```python
from build123d import *

# Parameters (mm, degrees)
BOSS_EXTRUDE1_DEPTH = 50
CUT_EXTRUDE1_DEPTH  = 50


with BuildPart() as part:
    # Sketch2 → Boss-Extrude1 (new body)
    with BuildSketch(Plane.XY):
        with BuildLine():
            Line((-133.871822526, 14.839434035), (-58.871822526, 14.839434035))
            Line((-58.871822526, 14.839434035), (15.717319626, 22.67906878))
            Line((15.717319626, 22.67906878), (16.762604259, 12.733849826))
            Line((16.762604259, 12.733849826), (-48.921026621, 5.830222033))
            ThreePointArc((-48.921026621, 5.830222033), (-58.375818015, -5.148257366), (-68.871822526, 4.839434035))
            Line((-68.871822526, 4.839434035), (-133.871822526, 4.839434035))
            Line((-133.871822526, 4.839434035), (-133.871822526, 14.839434035))
        make_face()
    extrude(amount=BOSS_EXTRUDE1_DEPTH)

    # Sketch4 → Cut-Extrude1 (cut)
    with BuildSketch(Plane.XY.offset(50)):
        with BuildLine():
            Line((-68.871822526, 0.839434035), (-68.871822526, 4.839434035))
            ThreePointArc((-68.871822526, 4.839434035), (-66.871822526, 2.839434035), (-68.871822526, 0.839434035))
        make_face()
        with BuildLine():
            Line((-48.502912768, 1.852134452), (-48.921026621, 5.830222033))
            ThreePointArc((-48.921026621, 5.830222033), (-50.701013486, 3.632121316), (-48.502912768, 1.852134452))
        make_face()
    extrude(amount=-CUT_EXTRUDE1_DEPTH, mode=Mode.SUBTRACT)


solid = part.part
```
Input: part model. Units: mm. Frame: model coordinates. A direction names the side the tool comes from. Coordinates: 2 decimals unless noted, no trailing zeros. Write each loop counter-clockwise with the first axis right and the second up, starting at its lowest first coordinate (ties: lowest second). Pieces come first, ordered by that corner, then holes. Notation, with made-up numbers: (79, 62) -> (106, 62) arc R14 cw to (106, 82) -> close; hole circle Ø10 at (-32.5, 63). An arc over 180 degrees is marked (long way). Answer as a JSON object with one key per item and string values.
1. First-contact query: P1, Ø4, axis at x = -63, z = 17, coming from the +Y side; P2, Ø4, axis at x = -32, z = 6.5, coming from the +Y side; P3, Ø3, axis at x = -1, z = 25, coming from the -Y side. Flat tips, straight axial feed; report the tip coordinate or a pass-through.
Result set:
{"P1": "stops at y = 14.84", "P2": "stops at y = 17.87", "P3": "stops at y = 10.71"}
2. Section B-B on x = -92. Return the cut outline in (y, z), then the cut area to 3 significant figures.
Result set:
{"outline": "(4.84, 0) -> (14.84, 0) -> (14.84, 50) -> (4.84, 50) -> close", "area": "500 mm2"}
3. Section C-C on y = 10.75. Return the cut outline in (x, z), then the cut area to 3 significant figures.
Result set:
{"outline": "(-133.87, 0) -> (-2.11, 0) -> (-2.11, 50) -> (-133.87, 50) -> close", "area": "6,590 mm2"}
4. Access query for faces 1 (the face through (-101, 4.839, 25)), 2 (the face through (-97, 14.839, 25)), 3 (the face through (-66.92, 3.27, 25.35)). Directions: +Z, -Z, +X, -X, +Y, -Y. A direction counts if a zero-diameter tool reaches every point of the face in a straight line with its end or side. Return the directions, or none.
Result set:
{"face 1": "+Z, -Z, -X, -Y", "face 2": "+Z, -Z, -X, +Y", "face 3": "+Z, -Z, -X"}
5. Section A-A on z = 7. Return the cut outline in (x, y).
Result set:
{"outline": "(-133.87, 4.84) -> (-68.87, 4.84) arc R2 cw to (-68.1, 0.99) arc R10 ccw to (-49.3, 1.93) arc R2 cw to (-48.92, 5.83) -> (16.76, 12.73) -> (15.72, 22.68) -> (-58.87, 14.84) -> (-133.87, 14.84) -> close"}
6. Material intervals for line 1 (Y direction, x = -99, z = 12.5); line 2 (X direction, y = 14, z = 14.5); line 3 (X direction, y = 2.25, z = 5), sorted ascending. Write a range as from..to.
Result set:
{"line 1": "y = 4.84..14.84", "line 2": "x = -133.87..16.63", "line 3": "x = -66.96..-49.92"}
